Can you work these out from the model? Positions are in its coordinate system, mm. A direction names the side the tool comes from. Coordinates: 2 decimals unless noted, no trailing zeros. Write each loop counter-clockwise with the first axis right and the second up, starting at its lowest first coordinate (ties: lowest second). Pieces come first, ordered by that corner, then holes. Notation, with made-up numbers: (-9.75, 64.25) -> (9.25, 64.25) arc R20 cw to (9.25, 100.25) -> close; hole circle Ø11 at (40, 27). An arc over 180 degrees is marked (long way). Use one line per item in the form item = value.
```python
from build123d import *

# Parameters (mm, degrees)
F0_R     = 2.5527
F0_R_2   = 4.7625
F1_DEPTH = 12


with BuildPart() as f1:
    # F0 (on Top) → F1 (new body)
    with BuildSketch(Plane.XY):
        with BuildLine():
            Line((274.091522, 50.8), (-259.308478, 50.8))
            Line((-259.308478, 50.8), (-259.308478, -152.4))
            Line((-259.308478, -152.4), (-462.508478, -152.4))
            Line((-462.508478, -152.4), (-462.508478, -177.8))
            Line((-462.508478, -177.8), (-208.508478, -177.8))
            Line((-208.508478, -177.8), (-208.508478, 0))
            Line((-208.508478, 0), (82.321522, 0))
            Line((82.321522, 0), (82.321522, -25.4))
            ThreePointArc((82.321522, -25.4), (107.721522, -50.8), (133.121522, -25.4))
            Line((133.121522, -25.4), (133.121522, 0))
            Line((133.121522, 0), (223.291522, 0))
            Line((223.291522, 0), (223.291522, -25.4))
            ThreePointArc((223.291522, -25.4), (248.691522, -50.8), (274.091522, -25.4))
            Line((274.091522, -25.4), (274.091522, 0))
            Line((274.091522, 0), (274.091522, 50.8))
        make_face()
        with Locations((-449.808478, -165.1)):
            Circle(F0_R, mode=Mode.SUBTRACT)
        with Locations((-424.408478, -165.1)):
            Circle(F0_R, mode=Mode.SUBTRACT)
        with Locations((-399.008478, -165.1)):
            Circle(F0_R, mode=Mode.SUBTRACT)
        with Locations((-373.608478, -165.1)):
            Circle(F0_R, mode=Mode.SUBTRACT)
        with Locations((-348.208478, -165.1)):
            Circle(F0_R, mode=Mode.SUBTRACT)
        with Locations((-322.808478, -165.1)):
            Circle(F0_R, mode=Mode.SUBTRACT)
        with Locations((-297.408478, -165.1)):
            Circle(F0_R, mode=Mode.SUBTRACT)
        with Locations((-272.008478, -165.1)):
            Circle(F0_R, mode=Mode.SUBTRACT)
        with Locations((-246.608478, -165.1)):
            Circle(F0_R, mode=Mode.SUBTRACT)
        with Locations((-221.208478, -165.1)):
            Circle(F0_R, mode=Mode.SUBTRACT)
        with Locations((-246.608478, -139.7)):
            Circle(F0_R, mode=Mode.SUBTRACT)
        with Locations((-221.208478, -139.7)):
            Circle(F0_R, mode=Mode.SUBTRACT)
        with Locations((-246.608478, -114.3)):
            Circle(F0_R, mode=Mode.SUBTRACT)
        with Locations((-221.208478, -114.3)):
            Circle(F0_R, mode=Mode.SUBTRACT)
        with Locations((-246.608478, -88.9)):
            Circle(F0_R, mode=Mode.SUBTRACT)
        with Locations((-221.208478, -88.9)):
            Circle(F0_R, mode=Mode.SUBTRACT)
        with Locations((-246.608478, -63.5)):
            Circle(F0_R, mode=Mode.SUBTRACT)
        with Locations((-221.208478, -63.5)):
            Circle(F0_R, mode=Mode.SUBTRACT)
        with Locations((-246.608478, -38.1)):
            Circle(F0_R, mode=Mode.SUBTRACT)
        with Locations((-221.208478, -38.1)):
            Circle(F0_R, mode=Mode.SUBTRACT)
        with Locations((-246.608478, -12.7)):
            Circle(F0_R, mode=Mode.SUBTRACT)
        with Locations((-221.208478, -12.7)):
            Circle(F0_R, mode=Mode.SUBTRACT)
        with Locations((-246.608478, 12.7)):
            Circle(F0_R, mode=Mode.SUBTRACT)
        with Locations((-221.208478, 12.7)):
            Circle(F0_R, mode=Mode.SUBTRACT)
        with Locations((-195.808478, 12.7)):
            Circle(F0_R, mode=Mode.SUBTRACT)
        with Locations((-170.408478, 12.7)):
            Circle(F0_R, mode=Mode.SUBTRACT)
        with Locations((-145.008478, 12.7)):
            Circle(F0_R, mode=Mode.SUBTRACT)
        with Locations((-119.608478, 12.7)):
            Circle(F0_R, mode=Mode.SUBTRACT)
        with Locations((-246.608478, 38.1)):
            Circle(F0_R, mode=Mode.SUBTRACT)
        with Locations((-221.208478, 38.1)):
            Circle(F0_R, mode=Mode.SUBTRACT)
        with Locations((-195.808478, 38.1)):
            Circle(F0_R, mode=Mode.SUBTRACT)
        with Locations((-170.408478, 38.1)):
            Circle(F0_R, mode=Mode.SUBTRACT)
        with Locations((-145.008478, 38.1)):
            Circle(F0_R, mode=Mode.SUBTRACT)
        with Locations((-119.608478, 38.1)):
            Circle(F0_R, mode=Mode.SUBTRACT)
        with Locations((107.721522, -25.4)):
            Circle(F0_R_2, mode=Mode.SUBTRACT)
        with Locations((248.691522, -25.4)):
            Circle(F0_R_2, mode=Mode.SUBTRACT)
        with Locations((-94.208478, 12.7)):
            Circle(F0_R, mode=Mode.SUBTRACT)
        with Locations((-68.808478, 12.7)):
            Circle(F0_R, mode=Mode.SUBTRACT)
        with Locations((-43.408478, 12.7)):
            Circle(F0_R, mode=Mode.SUBTRACT)
        with Locations((-18.008478, 12.7)):
            Circle(F0_R, mode=Mode.SUBTRACT)
        with Locations((7.391522, 12.7)):
            Circle(F0_R, mode=Mode.SUBTRACT)
        with Locations((32.791522, 12.7)):
            Circle(F0_R, mode=Mode.SUBTRACT)
        with Locations((58.191522, 12.7)):
            Circle(F0_R, mode=Mode.SUBTRACT)
        with Locations((83.591522, 12.7)):
            Circle(F0_R, mode=Mode.SUBTRACT)
        with Locations((-94.208478, 38.1)):
            Circle(F0_R, mode=Mode.SUBTRACT)
        with Locations((-68.808478, 38.1)):
            Circle(F0_R, mode=Mode.SUBTRACT)
        with Locations((-43.408478, 38.1)):
            Circle(F0_R, mode=Mode.SUBTRACT)
        with Locations((-18.008478, 38.1)):
            Circle(F0_R, mode=Mode.SUBTRACT)
        with Locations((7.391522, 38.1)):
            Circle(F0_R, mode=Mode.SUBTRACT)
        with Locations((32.791522, 38.1)):
            Circle(F0_R, mode=Mode.SUBTRACT)
        with Locations((58.191522, 38.1)):
            Circle(F0_R, mode=Mode.SUBTRACT)
        with Locations((83.591522, 38.1)):
            Circle(F0_R, mode=Mode.SUBTRACT)
        with Locations((108.991522, 12.7)):
            Circle(F0_R, mode=Mode.SUBTRACT)
        with Locations((134.391522, 12.7)):
            Circle(F0_R, mode=Mode.SUBTRACT)
        with Locations((159.791522, 12.7)):
            Circle(F0_R, mode=Mode.SUBTRACT)
        with Locations((185.191522, 12.7)):
            Circle(F0_R, mode=Mode.SUBTRACT)
        with Locations((210.591522, 12.7)):
            Circle(F0_R, mode=Mode.SUBTRACT)
        with Locations((235.991522, 12.7)):
            Circle(F0_R, mode=Mode.SUBTRACT)
        with Locations((261.391522, 12.7)):
            Circle(F0_R, mode=Mode.SUBTRACT)
        with Locations((108.991522, 38.1)):
            Circle(F0_R, mode=Mode.SUBTRACT)
        with Locations((134.391522, 38.1)):
            Circle(F0_R, mode=Mode.SUBTRACT)
        with Locations((159.791522, 38.1)):
            Circle(F0_R, mode=Mode.SUBTRACT)
        with Locations((185.191522, 38.1)):
            Circle(F0_R, mode=Mode.SUBTRACT)
        with Locations((210.591522, 38.1)):
            Circle(F0_R, mode=Mode.SUBTRACT)
        with Locations((235.991522, 38.1)):
            Circle(F0_R, mode=Mode.SUBTRACT)
        with Locations((261.391522, 38.1)):
            Circle(F0_R, mode=Mode.SUBTRACT)
    extrude(amount=F1_DEPTH)


solid = f1.part
```
Q1. If I drill on line 1 (X direction, y = -139.7, z = 9.25); line 2 (X direction, y = -6.5, z = 9); line 3 (X direction, y = -24, z = 5), over which ranges is the centre line in solid material (lowest first)? Write a range as from..to.
Return value:
line_1 = -259.31..-249.16, -244.06..-223.76, -218.66..-208.51
line_2 = -259.31..-208.51, 82.32..133.12, 223.29..274.09
line_3 = -259.31..-208.51, 82.32..103.17, 112.27..133.12, 223.29..244.14, 253.24..274.09
Q2. Thinking about a two-plate mould opening in X: for faces 1 (the flat face through (178, 0, 6)), 2 (the flat face through (274.092, 12, 6)), 3 (the flat face through (-41, 5, 12)), which applies, released by +X, released by -X, zero draft, split by the parting line, or undercut?
Return value:
face_1 = undercut
face_2 = released by +X
face_3 = zero draft
Q3. For faces 4 (the flat face through (82.322, -13, 6)), 5 (the flat face through (-41, 5, 0)), 6 (the flat face through (-259.308, -49, 6)), which set-ups out of +Z, -Z, +X, -X, +Y, -Y let a thin tool reach every point of the face, with its end or its side?
Return value:
face_4 = +Z, -Z, -Y
face_5 = -Z, +X, -X, +Y, -Y
face_6 = +Z, -Z, -X, +Y
Q4. Suppose I cut it at A-A (z = 3.5). Give the number of separate pieces and of enclosed holes in the cut face, then the cut area to 3 significant figures.
Return value:
separate_pieces = 1
enclosed_holes = 66
area = 44,400 mm2
Q5. Suppose I cut it at B-B (x = -414). Write out the boundary of the cut face in (y, z), then the cut area to 3 significant figures.
Return value:
outline = (-177.8, 0) -> (-152.4, 0) -> (-152.4, 12) -> (-177.8, 12) -> close
area = 305 mm2
Q6. Will these pins go through, and if not, where does the flat tip stop? pin 1 (1.5 mm diameter, centred on x = -117.5, z = 8, fed in from -Y); pin 2 (3 mm diameter, centred on y = -10, z = 2.5, fed in from -X); pin 3 (5 mm diameter, centred on x = 108.5, z = 4, fed in from -Y).
Return value:
pin_1 = 0
pin_2 = -259.31
pin_3 = -50.8
